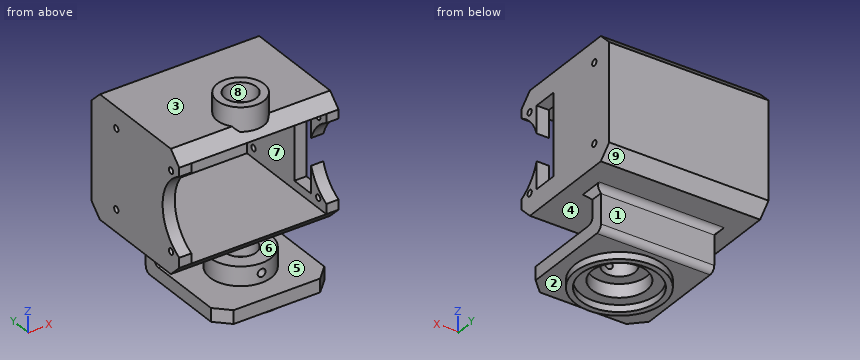
from build123d import *

# Parameters (mm, degrees)
SKETCH1_W                       = 25
SKETCH1_H                       = 30
BOSS_EXTRUDE1_DEPTH             = 3.175
SKETCH2_W                       = 25
SKETCH2_H                       = 3.175
BOSS_EXTRUDE2_DEPTH             = 41.58
SKETCH3_W                       = 3.175
SKETCH3_H                       = 25
BOSS_EXTRUDE3_DEPTH             = 30
CUT_EXTRUDE1_REACH              = 60.775
SKETCH4_R                       = 11.5
CUT_EXTRUDE2_REACH              = 60.775
SKETCH5_R                       = 0.8
CUT_EXTRUDE3_REACH              = 60.775
SKETCH6_R                       = 0.8
SKETCH6_R_2                     = 0.799851166
SKETCH6_W                       = 21.2
SKETCH6_H                       = 6.375
CUT_EXTRUDE4_REACH              = 60.775
SKETCH7_R                       = 11.5
BOSS_EXTRUDE4_DEPTH             = 0.2
SKETCH9_W                       = 41.58
SKETCH9_H                       = 33.175
BOSS_EXTRUDE5_DEPTH             = 3.175
BOSS_EXTRUDE6_DEPTH             = 0.2
SKETCH11_W                      = 41.58
SKETCH11_H                      = 33.175
BOSS_EXTRUDE7_DEPTH             = 3.175
CHAMFER1_SIZE                   = 3.175
CHAMFER2_SIZE                   = 3.175
SKETCH13_W                      = 29.58
SKETCH13_H                      = 3.175
BOSS_EXTRUDE8_DEPTH             = 7.695
BOSS_EXTRUDE9_REACH             = 59.968
SKETCH14_W                      = 29.58
SKETCH14_H                      = 3.5
BOSS_EXTRUDE9_DIRECTION_2_DEPTH = 25
CHAMFER3_SIZE                   = 3.5
FILLET1_R                       = 1.5875
FILLET2_R                       = 1.5875
CUT_EXTRUDE5_REACH              = 70.161
SKETCH16_R                      = 7.1
SKETCH20_R                      = 8
SKETCH20_R_2                    = 4.1
BOSS_EXTRUDE11_DEPTH            = 5
CUT_EXTRUDE6_START              = -21.7275
SKETCH21_R                      = 1.025
CUT_EXTRUDE6_DEPTH              = 16
BOSS_EXTRUDE12_DEPTH            = 5
BOSS_EXTRUDE12_DEPTH_BACK       = 1.2
SKETCH23_R                      = 6.1
SKETCH23_R_2                    = 4.1
CHAMFER4_SIZE                   = 1.5
SKETCH24_R                      = 11.5
SKETCH24_R_2                    = 10
BOSS_EXTRUDE13_DEPTH            = 1.8


with BuildPart() as part:
    # Sketch1 → Boss-Extrude1 (new body)
    with BuildSketch(Plane(origin=(0, 0, 0), x_dir=(0, 0, -1), z_dir=(1, 0, 0))):
        with Locations((12.5, 15)):
            Rectangle(SKETCH1_W, SKETCH1_H)
    extrude(amount=BOSS_EXTRUDE1_DEPTH)

    # Sketch2 → Boss-Extrude2 (add)
    with BuildSketch(Plane.ZY):
        with Locations((-12.5, 31.5875)):
            Rectangle(SKETCH2_W, SKETCH2_H)
    extrude(amount=-BOSS_EXTRUDE2_DEPTH)

    # Sketch3 → Boss-Extrude3 (add)
    with BuildSketch(Plane.XZ.offset(-30)):
        with Locations((39.9925, -12.5)):
            Rectangle(SKETCH3_W, SKETCH3_H)
    extrude(amount=BOSS_EXTRUDE3_DEPTH)

    # Sketch4 → Cut-Extrude1 (cut, up to next)
    with BuildSketch(Plane.ZY, mode=Mode.PRIVATE) as cut_extrude1_sk1:
        with Locations((-12.359999929, -5.209996254)):
            Circle(SKETCH4_R)
    cut_extrude1_tool1 = extrude(cut_extrude1_sk1.sketch, amount=-CUT_EXTRUDE1_REACH, mode=Mode.PRIVATE) & part.part
    add(cut_extrude1_tool1.solids().sort_by_distance((0, -5.209996, -12.36))[0], mode=Mode.SUBTRACT)

    # Sketch5 → Cut-Extrude2 (cut, up to next)
    with BuildSketch(Plane.ZY, mode=Mode.PRIVATE) as cut_extrude2_sk1:
        with Locations((-22.609999929, 3.090003746)):
            Circle(SKETCH5_R)
    cut_extrude2_tool1 = extrude(cut_extrude2_sk1.sketch, amount=-CUT_EXTRUDE2_REACH, mode=Mode.PRIVATE) & part.part
    # Sketch5 → Cut-Extrude2 (cut, up to next)
    with BuildSketch(Plane.ZY, mode=Mode.PRIVATE) as cut_extrude2_sk2:
        with Locations((-22.609999929, 23.790003746)):
            Circle(SKETCH5_R)
    cut_extrude2_tool2 = extrude(cut_extrude2_sk2.sketch, amount=-CUT_EXTRUDE2_REACH, mode=Mode.PRIVATE) & part.part
    # Sketch5 → Cut-Extrude2 (cut, up to next)
    with BuildSketch(Plane.ZY, mode=Mode.PRIVATE) as cut_extrude2_sk3:
        with Locations((-2.109999929, 23.790003746)):
            Circle(SKETCH5_R)
    cut_extrude2_tool3 = extrude(cut_extrude2_sk3.sketch, amount=-CUT_EXTRUDE2_REACH, mode=Mode.PRIVATE) & part.part
    # Sketch5 → Cut-Extrude2 (cut, up to next)
    with BuildSketch(Plane.ZY, mode=Mode.PRIVATE) as cut_extrude2_sk4:
        with Locations((-2.109999929, 3.090003746)):
            Circle(SKETCH5_R)
    cut_extrude2_tool4 = extrude(cut_extrude2_sk4.sketch, amount=-CUT_EXTRUDE2_REACH, mode=Mode.PRIVATE) & part.part
    add(cut_extrude2_tool1.solids().sort_by_distance((0, 3.090004, -22.61))[0], mode=Mode.SUBTRACT)
    add(cut_extrude2_tool2.solids().sort_by_distance((0, 23.790004, -22.61))[0], mode=Mode.SUBTRACT)
    add(cut_extrude2_tool3.solids().sort_by_distance((0, 23.790004, -2.11))[0], mode=Mode.SUBTRACT)
    add(cut_extrude2_tool4.solids().sort_by_distance((0, 3.090004, -2.11))[0], mode=Mode.SUBTRACT)

    # Sketch6 → Cut-Extrude3 (cut, up to next)
    with BuildSketch(Plane(origin=(41.58, 0, 0), x_dir=(0, 0, -1), z_dir=(1, 0, 0)), mode=Mode.PRIVATE) as cut_extrude3_sk1:
        with Locations(Location((2.109999929, 3.090003746, 0), (0, 0, 180))):
            Circle(SKETCH6_R)
    cut_extrude3_tool1 = extrude(cut_extrude3_sk1.sketch, amount=-CUT_EXTRUDE3_REACH, mode=Mode.PRIVATE) & part.part
    # Sketch6 → Cut-Extrude3 (cut, up to next)
    with BuildSketch(Plane(origin=(41.58, 0, 0), x_dir=(0, 0, -1), z_dir=(1, 0, 0)), mode=Mode.PRIVATE) as cut_extrude3_sk2:
        with Locations(Location((22.609999929, 3.090003746, 0), (0, 0, 180))):
            Circle(SKETCH6_R)
    cut_extrude3_tool2 = extrude(cut_extrude3_sk2.sketch, amount=-CUT_EXTRUDE3_REACH, mode=Mode.PRIVATE) & part.part
    # Sketch6 → Cut-Extrude3 (cut, up to next)
    with BuildSketch(Plane(origin=(41.58, 0, 0), x_dir=(0, 0, -1), z_dir=(1, 0, 0)), mode=Mode.PRIVATE) as cut_extrude3_sk3:
        with Locations((22.609999929, 27.540003746)):
            Circle(SKETCH6_R_2)
    cut_extrude3_tool3 = extrude(cut_extrude3_sk3.sketch, amount=-CUT_EXTRUDE3_REACH, mode=Mode.PRIVATE) & part.part
    # Sketch6 → Cut-Extrude3 (cut, up to next)
    with BuildSketch(Plane(origin=(41.58, 0, 0), x_dir=(0, 0, -1), z_dir=(1, 0, 0)), mode=Mode.PRIVATE) as cut_extrude3_sk4:
        with Locations((2.109999929, 27.540003746)):
            Circle(SKETCH6_R)
    cut_extrude3_tool4 = extrude(cut_extrude3_sk4.sketch, amount=-CUT_EXTRUDE3_REACH, mode=Mode.PRIVATE) & part.part
    # Sketch6 → Cut-Extrude3 (cut, up to next)
    with BuildSketch(Plane(origin=(41.58, 0, 0), x_dir=(0, 0, -1), z_dir=(1, 0, 0)), mode=Mode.PRIVATE) as cut_extrude3_sk5:
        with Locations((12.359999929, 8.927503746)):
            Rectangle(SKETCH6_W, SKETCH6_H)
    cut_extrude3_tool5 = extrude(cut_extrude3_sk5.sketch, amount=-CUT_EXTRUDE3_REACH, mode=Mode.PRIVATE) & part.part
    add(cut_extrude3_tool1.solids().sort_by_distance((41.58, 3.090004, -2.11))[0], mode=Mode.SUBTRACT)
    add(cut_extrude3_tool2.solids().sort_by_distance((41.58, 3.090004, -22.61))[0], mode=Mode.SUBTRACT)
    add(cut_extrude3_tool3.solids().sort_by_distance((41.58, 27.540004, -22.61))[0], mode=Mode.SUBTRACT)
    add(cut_extrude3_tool4.solids().sort_by_distance((41.58, 27.540004, -2.11))[0], mode=Mode.SUBTRACT)
    add(cut_extrude3_tool5.solids().sort_by_distance((41.58, 8.927504, -12.36))[0], mode=Mode.SUBTRACT)

    # Sketch7 → Cut-Extrude4 (cut, up to next)
    with BuildSketch(Plane(origin=(41.58, 0, 0), x_dir=(0, 0, -1), z_dir=(1, 0, 0)), mode=Mode.PRIVATE) as cut_extrude4_sk1:
        with Locations((12.359999929, -5.209996254)):
            Circle(SKETCH7_R)
    cut_extrude4_tool1 = extrude(cut_extrude4_sk1.sketch, amount=-CUT_EXTRUDE4_REACH, mode=Mode.PRIVATE) & part.part
    add(cut_extrude4_tool1.solids().sort_by_distance((41.58, -5.209996, -12.36))[0], mode=Mode.SUBTRACT)

    # Sketch8 → Boss-Extrude4 (add)
    with BuildSketch(Plane.XY):
        Polygon((0, 33.175), (0, 0), (3.175, 0), (3.175, 30), (38.405, 30), (38.405, 0), (41.58, 0), (41.58, 33.175), align=None)
    extrude(amount=BOSS_EXTRUDE4_DEPTH)

    # Sketch9 → Boss-Extrude5 (add)
    with BuildSketch(Plane.XY.offset(0.2)):
        with Locations((20.79, 16.5875)):
            Rectangle(SKETCH9_W, SKETCH9_H)
    extrude(amount=BOSS_EXTRUDE5_DEPTH)

    # Sketch10 → Boss-Extrude6 (add)
    with BuildSketch(Plane(origin=(0, 0, -25), x_dir=(-1, 0, 0), z_dir=(0, 0, -1))):
        Polygon((0, 0), (0, 33.175), (-41.58, 33.175), (-41.58, 0), (-38.405, 0), (-38.405, 30), (-3.175, 30), (-3.175, 0), align=None)
    extrude(amount=BOSS_EXTRUDE6_DEPTH)

    # Sketch11 → Boss-Extrude7 (add)
    with BuildSketch(Plane(origin=(0, 0, -25.2), x_dir=(-1, 0, 0), z_dir=(0, 0, -1))):
        with Locations((-20.79, 16.5875)):
            Rectangle(SKETCH11_W, SKETCH11_H)
    extrude(amount=BOSS_EXTRUDE7_DEPTH)

    # Chamfer1
    chamfer1_edges = [part.edges().sort_by_distance(p)[0] for p in [
        (20.79, 33.175, 3.375),
        (20.79, 33.175, -28.375),
    ]]
    chamfer(chamfer1_edges, length=CHAMFER1_SIZE)

    # Chamfer2
    chamfer2_edges = [part.edges().sort_by_distance(p)[0] for p in [
        (20.79, 0, 3.375),
        (20.79, 0, -28.375),
    ]]
    chamfer(chamfer2_edges, length=CHAMFER2_SIZE - 0.0001)  # a hair under: the kernel refuses the full size

    # Sketch13 → Boss-Extrude8 (add)
    with BuildSketch(Plane(origin=(0, 0, -28.375), x_dir=(-1, 0, 0), z_dir=(0, 0, -1))):
        with Locations((-20.79, 19.7625)):
            Rectangle(SKETCH13_W, SKETCH13_H)
    extrude(amount=BOSS_EXTRUDE8_DEPTH)

    # Boss-Extrude9: up to this face of the body (flat: up to its plane)
    boss_extrude9_end = Plane(part.part.faces().sort_by_distance((20.79, 21.35, -32.2225))[0])
    # Sketch14 → Boss-Extrude9 (add, up to the picked face)
    with BuildSketch(Plane.XZ.offset(-18.175), mode=Mode.PRIVATE) as boss_extrude9_sk1:
        with Locations((20.79, -37.495)):
            Rectangle(SKETCH14_W, SKETCH14_H)
    boss_extrude9_tool1 = split(extrude(boss_extrude9_sk1.sketch, amount=-BOSS_EXTRUDE9_REACH, mode=Mode.PRIVATE), bisect_by=boss_extrude9_end, keep=Keep.BOTH, mode=Mode.PRIVATE)
    add(boss_extrude9_tool1.solids().sort_by(Axis((20.79, 18.175, -37.495), (0, 1, 0)))[0])

    # Sketch14 → Boss-Extrude9 direction 2 (add)
    with BuildSketch(Plane.XZ.offset(-18.175)):
        with Locations((20.79, -37.495)):
            Rectangle(SKETCH14_W, SKETCH14_H)
    extrude(amount=BOSS_EXTRUDE9_DIRECTION_2_DEPTH)

    # Chamfer3
    chamfer3_edges = [part.edges().sort_by_distance(p)[0] for p in [
        (6, -6.825, -37.495),
        (35.58, -6.825, -37.495),
    ]]
    chamfer(chamfer3_edges, length=CHAMFER3_SIZE)

    # Fillet1
    fillet1_edges = [part.edges().sort_by_distance(p)[0] for p in [
        (20.79, 18.175, -35.745),
        (20.79, 21.35, -39.245),
    ]]
    fillet(fillet1_edges, radius=FILLET1_R)

    # Fillet2
    fillet2_edges = [part.edges().sort_by_distance(p)[0] for p in [
        (20.79, 21.35, -28.375),
    ]]
    fillet(fillet2_edges, radius=FILLET2_R)

    # Sketch16 → Cut-Extrude5 (cut, up to next)
    with BuildSketch(Plane(origin=(0, 0, -39.245), x_dir=(-1, 0, 0), z_dir=(0, 0, -1)), mode=Mode.PRIVATE) as cut_extrude5_sk1:
        with Locations((-20.79, 6.9025)):
            Circle(SKETCH16_R)
    cut_extrude5_tool1 = extrude(cut_extrude5_sk1.sketch, amount=-CUT_EXTRUDE5_REACH, mode=Mode.PRIVATE) & part.part
    add(cut_extrude5_tool1.solids().sort_by_distance((20.79, 6.9025, -39.245))[0], mode=Mode.SUBTRACT)

    # Sketch20 → Boss-Extrude11 (add)
    with BuildSketch(Plane.XY.offset(-35.745)):
        with Locations(Location((20.79, 6.9025, 0), (0, 0, 180))):
            Circle(SKETCH20_R)
        with Locations((20.79, 6.9025)):
            Circle(SKETCH20_R_2, mode=Mode.SUBTRACT)
    extrude(amount=BOSS_EXTRUDE11_DEPTH)

    # Sketch21 → Cut-Extrude6 (cut)
    with BuildSketch(Plane.XZ.offset(6.825).offset(CUT_EXTRUDE6_START)):
        with Locations(Location((20.79, -33.245, 0), (0, 0, 270))):
            Circle(SKETCH21_R)
    extrude(amount=CUT_EXTRUDE6_DEPTH, mode=Mode.SUBTRACT)

    # Sketch23 → Boss-Extrude12 (add, two sides: drawn at the far end of the back side and taken through both)
    with BuildSketch(Plane.XY.offset(3.375).offset(-BOSS_EXTRUDE12_DEPTH_BACK)):
        with Locations(Location((20.79, 6.9025, 0), (0, 0, 217.666590828))):
            Circle(SKETCH23_R)
        with Locations((20.79, 6.9025)):
            Circle(SKETCH23_R_2, mode=Mode.SUBTRACT)
    extrude(amount=BOSS_EXTRUDE12_DEPTH + BOSS_EXTRUDE12_DEPTH_BACK)

    # Chamfer4
    chamfer4_edges = [part.edges().sort_by_distance(p)[0] for p in [
        (35.58, 20.55625, -28.375),
        (20.79, 18.175, -28.375),
        (6, 20.55625, -28.375),
    ]]
    chamfer(chamfer4_edges, length=CHAMFER4_SIZE)

    # Sketch24 → Boss-Extrude13 (add)
    with BuildSketch(Plane(origin=(0, 0, -39.245), x_dir=(-1, 0, 0), z_dir=(0, 0, -1))):
        with Locations(Location((-20.79, 6.9025, 0), (0, 0, 180))):
            Circle(SKETCH24_R)
        with Locations((-20.79, 6.9025)):
            Circle(SKETCH24_R_2, mode=Mode.SUBTRACT)
    extrude(amount=BOSS_EXTRUDE13_DEPTH)


solid = part.part
Here's how the part is built. I have some questions about the finished solid (model axes, mm). Face numbers are marked on the shaded views. A direction names the side the tool comes from. Give positions to 0.01 mm unless a question says otherwise; leave off trailing zeros. Write each loop counter-clockwise with the first axis right and the second up, starting at its lowest first coordinate (ties: lowest second). Pieces come first, ordered by that corner, then holes. Notation, with made-up numbers: (83, 81.25) -> (141, 81.25) arc R37 ccw to (141, 120.25) -> close; hole circle Ø4 at (7, -10.75). An arc over 180 degrees is marked (long way). Use one line per item in the form item = value. Start each with the question number.
1. Will these pins go through, and if not, where does the flat tip stop? pin 1 Ø5 at (x, y) = (35.5, 21) entering from -Z (3 decimals); pin 2 Ø7 at (x, y) = (17.5, 6) entering from -Z (3 decimals); pin 3 Ø5 at (x, y) = (11, 6) entering from +Z (3 decimals).
2. Imagine slicing it at D-D on z = -17. List the corners of the cut face in (x, y) for me (3 decimals), plus the area to 3 significant figures.
3. On a 3-axis mill with a long thin cutter (end or side, diameter ignored), from which of +Z, -Z, +X, -X, +Y, -Y can I reach the whole of each face in a straight line? I mean the marked faces 5, 6, 7, 8 and 9. Say none if no direction works.
4. Imagine slicing it at A-A on z = -8. List the corners of the cut face in (x, y) for me (3 decimals).
5. If I drill on L1, parallel to Y at x = 1.6, z = -2.11 (3 decimals); L2, parallel to Z at x = 26.5, y = 16.5 (3 decimals); L3, parallel to X at y = 6.5, z = -37, over which ranges is the centre line in solid material (lowest first)?
6. Imagine slicing it at B-B on x = 20.79. State how many separate pieces and enclosed holes the cut face has, plus the area to 3 significant figures.
7. Thinking about a two-plate mould opening in Z: for the marked faces 1, 2, 3 and 4, which applies, +Z half, -Z half, draft (parallel to the pull), parting line (faces both ways), or undercut?
Entries:
q1.pin_1 = -39.245
q1.pin_2 = -35.745
q1.pin_3 = 3.375
q2.outline = (0, 5.312) -> (3.175, 5.312) -> (3.175, 30) -> (38.405, 30) -> (38.405, 12.115) -> (41.58, 12.115) -> (41.58, 33.175) -> (0, 33.175) -> close; (38.405, 5.312) -> (41.58, 5.312) -> (41.58, 5.74) -> (38.405, 5.74) -> close
q2.area = 269 mm²
q3.face_5 = none
q3.face_6 = +X, -X, -Y
q3.face_7 = -Y
q3.face_8 = +Z
q3.face_9 = -Z, +X, -X, +Y
q4.outline = (0, 5.431) -> (3.175, 5.431) -> (3.175, 30) -> (38.405, 30) -> (38.405, 12.115) -> (41.58, 12.115) -> (41.58, 33.175) -> (0, 33.175) -> close; (38.405, 5.431) -> (41.58, 5.431) -> (41.58, 5.74) -> (38.405, 5.74) -> close
q5.L1 = 0.004 to 2.29, 3.89 to 22.99, 24.59 to 33.175
q5.L2 = -41.045 to -35.745, -28.375 to -25.2, 0.2 to 3.375
q5.L3 = 6 to 13.7, 27.88 to 35.58
q6.separate_pieces = 4
q6.enclosed_holes = 0
q6.area = 396 mm²
q7.face_1 = draft
q7.face_2 = -Z half
q7.face_3 = +Z half
q7.face_4 = undercut
